Part model, mm, in its own coordinate system. Face numbers are marked on the shaded views. A direction names the side the tool comes from. Round coordinates to 2 decimals unless told otherwise and drop trailing zeros. Loops run counter-clockwise (first coordinate to the right, second up) from the corner with the lowest first, then second, coordinate; pieces in that order, holes last. Notation, with made-up numbers: M 4.25,-17.5 L 34.25,-17.5 A18 ccw 34.25,-2.5 Z; hole C -21,89.5 d5. An arc over 180 degrees is marked long. Put each result on its own line as item: value. Start each with the question number.
```python
from build123d import *

# Parameters (mm, degrees)
F0_W     = 84
F0_H     = 84
F1_DEPTH = 4
F2_W     = 7.5
F2_H     = 1
F3_DEPTH = 8.5
F4_R     = 1
F5_DEPTH = 25
F6_START = -2
F4_R_2   = 1.5
F6_DEPTH = 23
F7_SIZE  = 1.5


with BuildPart() as f1:
    # F0 (on Top) → F1 (new body)
    with BuildSketch(Plane.XY):
        Rectangle(F0_W, F0_H)
    extrude(amount=F1_DEPTH)

    # F2 (on face) → F3 (join)
    with BuildSketch(Plane.XY.offset(4)):
        Polygon((-30, 27), (-32, 27), (-32, 24.5), (-30, 24.5), (-30, 25.5), (-30.75, 25.5), (-30.75, 26), (-30, 26), align=None)
        with Locations((-26.25, 26.5)):
            Rectangle(F2_W, F2_H)
        Polygon((-20.5, 27), (-22.5, 27), (-22.5, 26), (-21.75, 26), (-21.75, 25.5), (-22.5, 25.5), (-22.5, 24.5), (-20.5, 24.5), align=None)
        Polygon((-32, -27), (-30, -27), (-30, -26), (-30.75, -26), (-30.75, -25.5), (-30, -25.5), (-30, -24.5), (-32, -24.5), align=None)
        with Locations((-26.25, -26.5)):
            Rectangle(F2_W, F2_H)
        Polygon((-22.5, -27), (-20.5, -27), (-20.5, -24.5), (-22.5, -24.5), (-22.5, -25.5), (-21.75, -25.5), (-21.75, -26), (-22.5, -26), align=None)
        Polygon((22.5, 27), (20.5, 27), (20.5, 24.5), (22.5, 24.5), (22.5, 25.5), (21.75, 25.5), (21.75, 26), (22.5, 26), align=None)
        with Locations((26.25, 26.5)):
            Rectangle(F2_W, F2_H)
        Polygon((32, 27), (30, 27), (30, 26), (30.75, 26), (30.75, 25.5), (30, 25.5), (30, 24.5), (32, 24.5), align=None)
        Polygon((20.5, -27), (22.5, -27), (22.5, -26), (21.75, -26), (21.75, -25.5), (22.5, -25.5), (22.5, -24.5), (20.5, -24.5), align=None)
        with Locations((26.25, -26.5)):
            Rectangle(F2_W, F2_H)
        Polygon((30, -27), (32, -27), (32, -24.5), (30, -24.5), (30, -25.5), (30.75, -25.5), (30.75, -26), (30, -26), align=None)
    extrude(amount=F3_DEPTH)

    # F4 (on face) → F5 (cut)
    with BuildSketch(Plane.XY.offset(4)):
        with Locations((0, 35)):
            Circle(F4_R)
    extrude(amount=-F5_DEPTH, mode=Mode.SUBTRACT)

    # F4 (on face) → F6 (cut)
    with BuildSketch(Plane.XY.offset(4).offset(F6_START)):
        with Locations((0, 35)):
            Circle(F4_R_2)
        with Locations((0, 35)):
            Circle(F4_R, mode=Mode.SUBTRACT)
    extrude(amount=-F6_DEPTH, mode=Mode.SUBTRACT)

    # F7
    f7_edges = [f1.edges().sort_by_distance(p)[0] for p in [
        (-1.5, 35, 0),
    ]]
    chamfer(f7_edges, length=F7_SIZE)


solid = f1.part
```
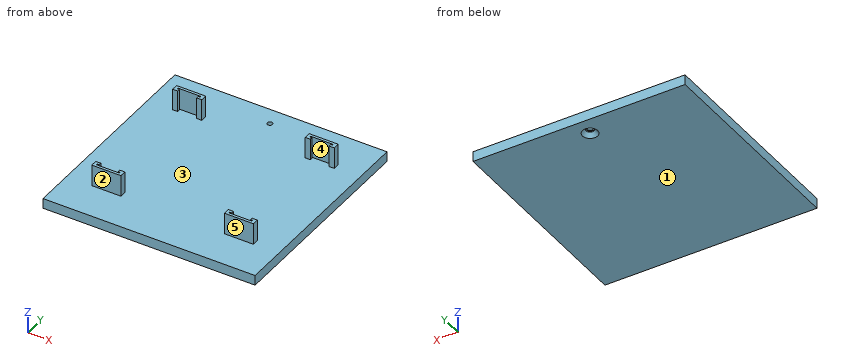
1. Cut at A-A, the plane x = 0. Give the cut face in (y, z), and give its area (3 significant figures).
2. Cut at C-C, the plane x = -26.5. Give the cut face in (y, z), and give its area (3 significant figures).
3. Mould opens along Y. For the marked faces 1, 2 and 3 say: released by +Y, released by -Y, zero draft, split by the parting line, or undercut.
4. Cut at D-D, the plane y = 1. Give the cut face in (x, z).
5. Which spindle directions (+Z, -Z, +X, -X, +Y, -Y) get a long thin tool onto all of the face, cutting with end or side? Do the marked faces 4 and 5. Say none if no direction does.
6. Drop flat-ended pins along their axis: pin 1 (0.8 mm diameter, centred on y = 25.5, z = 7.5, fed in from +X); pin 2 (3 mm diameter, centred on x = 19.5, z = 10, fed in from -Y); pin 3 (0.8 mm diameter, centred on x = -30, z = 10, fed in from +Y). Give the stop position or say it passes through.
7. Wall check: L1, parallel to Y at x = 0, z = 3.3; L2, parallel to Z at x = 23, y = 6.5; L3, parallel to Y at x = -0.5, z = 1.25. Give the ranges that are in metal, low to high.
8. Cut at B-B, the plane y = 35. Give the cut face in (x, z).
Results list:
1. outline: M -42,0 L 32,0 L 33.5,1.5 L 33.5,2 L 34,2 L 34,4 L -42,4 Z; M 36,2 L 36.5,2 L 36.5,1.5 L 38,0 L 42,0 L 42,4 L 36,4 Z
1. area: 324 mm^2
2. outline: M -42,0 L 42,0 L 42,4 L 27,4 L 27,12.5 L 26,12.5 L 26,4 L -26,4 L -26,12.5 L -27,12.5 L -27,4 L -42,4 Z
2. area: 353 mm^2
3. face 1: zero draft
3. face 2: released by -Y
3. face 3: undercut
4. outline: M -42,0 L 42,0 L 42,4 L -42,4 Z
5. face 4: +Z
5. face 5: +Z, +X, -X, -Y
6. pin 1: stops at x = 32
6. pin 2: stops at y = -27
6. pin 3: stops at y = 27
7. L1: y = -42 to 34, 36 to 42
7. L2: z = 0 to 4
7. L3: y = -42 to 33.32, 36.68 to 42
8. outline: M -42,0 L -3,0 L -1.5,1.5 L -1.5,2 L -1,2 L -1,4 L -42,4 Z; M 1,2 L 1.5,2 L 1.5,1.5 L 3,0 L 42,0 L 42,4 L 1,4 Z
